Model file for the job. Use its own axes, mm. A direction names the side the tool comes from. Round coordinates to 2 decimals unless told otherwise and drop trailing zeros. Loops run counter-clockwise (first coordinate to the right, second up) from the corner with the lowest first, then second, coordinate; pieces in that order, holes last. Notation, with made-up numbers: M -24,-28.5 L 0,-28.5 A4 cw 0,-22.5 Z; hole C -7.75,-23.75 d3. An arc over 180 degrees is marked long. Use a Markdown table: item, result. Add a question column.
Item 1: Wall check: L1, parallel to X at y = 1.25, z = -7.5; L2, parallel to Y at x = 3, z = -8; L3, parallel to X at y = -25, z = -2. Give the ranges that are in metal, low to high. Write a range as from..to.
Item 2: Saw through at B-B on y = -9.5. Write the cut outline in (x, z).
Item 3: Saw through at A-A on x = -17.5. Write the cut outline in (y, z).
Item 4: Saw through at C-C on z = 0.25. Write the cut outline in (x, y).
Item 5: Two-plate mould, pull along Z, no slides. Class faces 4 (the flat face through (3, -30, -9.15)), 5 (the flat face through (3, -30, 9.15)), 6 (the cylindrical face through (-21.9, 1.52, 11.93)), 7 (the flat face through (-15, 0, 0)): +Z half, -Z half, draft (parallel to the pull), parting line (faces both ways), or undercut.
Item 6: Saw through at D-D on x = 13. Write the cut outline in (y, z).
Item 7: Pin check, flat tips, straight feed: P1, Ø4.5, axis at x = 17.5, z = 7.5, coming from the +Y side; P2, Ø3.5, axis at y = -31.5, z = -3.5, coming from the -X side; P3, Ø1.7, axis at y = -29, z = 7, coming from the +X side; P4, Ø1.5, axis at y = -19, z = -6.5, coming from the +X side. Stop position of each tip, or through.
Item 8: Tool access for faces 1 (the flat face through (2.5, -32, -5)), 2 (the cylindrical face through (-5.227, -4.803, 0.175)), 3 (the cylindrical face through (5.227, -4.803, 0.175)): list every direction of +Z, -Z, +X, -X, +Y, -Y with a clear straight run to the whole face (end or side of a thin tool).
```python
from build123d import *

# Parameters (mm, degrees)
SKETCH1_W           = 45
SKETCH1_H           = 25
SKETCH1_R           = 1.7
BOSS_EXTRUDE1_DEPTH = 3
SKETCH2_W           = 10
SKETCH2_H           = 25
BOSS_EXTRUDE2_DEPTH = 5
BOSS_EXTRUDE3_DEPTH = 25
CUT_EXTRUDE1_DEPTH  = 50.590533486
SKETCH5_R           = 1.7
CUT_EXTRUDE2_DEPTH  = 47.75971569
CUT_EXTRUDE3_DEPTH  = 1.5
FILLET1_R           = 2
FILLET2_R           = 2
FILLET3_R           = 2


with BuildPart() as part:
    # Sketch1 → Boss-Extrude1 (new body)
    with BuildSketch(Plane(origin=(0, 0, 0), x_dir=(1, 0, 0), z_dir=(0, 1, 0))):
        Rectangle(SKETCH1_W, SKETCH1_H)
        with Locations(Location((-17.5, 7.5, 0), (0, 0, 270))):
            Circle(SKETCH1_R, mode=Mode.SUBTRACT)
        with Locations(Location((17.5, 7.5, 0), (0, 0, 270))):
            Circle(SKETCH1_R, mode=Mode.SUBTRACT)
        with Locations(Location((17.5, -7.5, 0), (0, 0, 270))):
            Circle(SKETCH1_R, mode=Mode.SUBTRACT)
        with Locations(Location((-17.5, -7.5, 0), (0, 0, 270))):
            Circle(SKETCH1_R, mode=Mode.SUBTRACT)
    extrude(amount=BOSS_EXTRUDE1_DEPTH)

    # Sketch2 → Boss-Extrude2 (add)
    with BuildSketch(Plane.XZ):
        Rectangle(SKETCH2_W, SKETCH2_H)
    extrude(amount=BOSS_EXTRUDE2_DEPTH)

    # Sketch3 → Boss-Extrude3 (add)
    with BuildSketch(Plane.XY.offset(12.5)):
        with BuildLine():
            Line((4, -23.941336576), (4, -36.441336576))
            Line((4, -36.441336576), (-4, -36.441336576))
            Line((-4, -36.441336576), (-4, -23.941336576))
            ThreePointArc((-4, -23.941336576), (-10.485397361, -14.786664856), (-5, -5))
            Line((-5, -5), (5, -5))
            ThreePointArc((5, -5), (10.485397361, -14.786664856), (4, -23.941336576))
        make_face()
    extrude(amount=-BOSS_EXTRUDE3_DEPTH)

    # Sketch4 → Cut-Extrude1 (cut, through all)
    with BuildSketch(Plane.XY.offset(12.5)):
        with BuildLine():
            Line((-0.75, -22.750134396), (-0.75, -36.441336576))
            Line((-0.75, -36.441336576), (0.75, -36.441336576))
            Line((0.75, -36.441336576), (0.75, -22.750134396))
            ThreePointArc((0.75, -22.750134396), (0, -5.683092656), (-0.75, -22.750134396))
        make_face()
    extrude(amount=-CUT_EXTRUDE1_DEPTH, mode=Mode.SUBTRACT)

    # Sketch5 → Cut-Extrude2 (cut, through all)
    with BuildSketch(Plane(origin=(4, 0, 0), x_dir=(0, 0, -1), z_dir=(1, 0, 0))):
        with Locations(Location((-6.25, -30.191336576, 0), (0, 0, 180))):
            Circle(SKETCH5_R)
        with Locations(Location((6.25, -30.191336576, 0), (0, 0, 180))):
            Circle(SKETCH5_R)
    extrude(amount=-CUT_EXTRUDE2_DEPTH, mode=Mode.SUBTRACT)

    # Sketch6 → Cut-Extrude3 (cut)
    with BuildSketch(Plane(origin=(4, 0, 0), x_dir=(0, 0, -1), z_dir=(1, 0, 0))):
        Polygon((9.15, -28.517020795), (6.25, -26.842705014), (3.35, -28.517020795), (3.35, -31.865652356), (6.25, -33.539968137), (9.15, -31.865652356), align=None)
        Polygon((-3.35, -28.517020795), (-6.25, -26.842705014), (-9.15, -28.517020795), (-9.15, -31.865652356), (-6.25, -33.539968137), (-3.35, -31.865652356), align=None)
    extrude(amount=-CUT_EXTRUDE3_DEPTH, mode=Mode.SUBTRACT)

    # Fillet1
    fillet1_edges = [part.edges().sort_by_distance(p)[0] for p in [
        (-22.5, 1.5, -12.5),
        (22.5, 1.5, -12.5),
        (22.5, 1.5, 12.5),
        (-22.5, 1.5, 12.5),
    ]]
    fillet(fillet1_edges, radius=FILLET1_R)

    # Fillet2
    fillet2_edges = [part.edges().sort_by_distance(p)[0] for p in [
        (-5, 0, 0),
        (5, 0, 0),
        (-5, -5, 0),
        (5, -5, 0),
    ]]
    fillet(fillet2_edges, radius=FILLET2_R)

    # Fillet3
    fillet3_edges = [part.edges().sort_by_distance(p)[0] for p in [
        (-2.375, -36.441336576, 12.5),
        (2.375, -36.441336576, -12.5),
        (-2.375, -36.441336576, -12.5),
        (2.375, -36.441336576, 12.5),
    ]]
    fillet(fillet3_edges, radius=FILLET3_R)


solid = part.part
```
Entries:
| question | item | result |
|---|---|---|
| 1 | L1 | -22.5..-19.2, -15.8..15.8, 19.2..22.5 |
| 1 | L2 | -36.44..-32.53, -27.85..-22.24, -6.23..3 |
| 1 | L3 | -4..-0.75, 0.75..4 |
| 2 | outline | M -9.37,-12.5 L -7.12,-12.5 L -7.12,12.5 L -9.37,12.5 Z; M 7.12,-12.5 L 9.37,-12.5 L 9.37,12.5 L 7.12,12.5 Z |
| 3 | outline | M 0,-12.5 L 3,-12.5 L 3,-9.2 L 0,-9.2 Z; M 0,-5.8 L 3,-5.8 L 3,5.8 L 0,5.8 Z; M 0,9.2 L 3,9.2 L 3,12.5 L 0,12.5 Z |
| 4 | outline | M -22.5,0 L -7,0 A2 cw -5,-2 L -5,-3.88 A2 cw -5.88,-5.53 A10.5 ccw -4,-23.94 L -4,-36.44 L -0.75,-36.44 L -0.75,-22.75 A8.55 cw long 0.75,-22.75 L 0.75,-36.44 L 4,-36.44 L 4,-23.94 A10.5 ccw 5.88,-5.53 A2 cw 5,-3.88 L 5,-2 A2 cw 7,0 L 22.5,0 L 22.5,3 L -22.5,3 Z |
| 5 | face 4 | undercut |
| 5 | face 5 | undercut |
| 5 | face 6 | +Z half |
| 5 | face 7 | draft |
| 6 | outline | M 0,-12.5 L 3,-12.5 L 3,12.5 L 0,12.5 Z |
| 7 | P1 | y = 3 |
| 7 | P2 | x = -4 |
| 7 | P3 | x = 2.5 |
| 7 | P4 | x = 9.7 |
| 8 | face 1 | +X |
| 8 | face 2 | +Z, -Z, -X |
| 8 | face 3 | +Z, -Z, +X |
